Source: three-view drawing plus pictorial views. Frame: mm from the lowest corner of the part. A direction names the side the tool comes from. Coordinates: 2 decimals unless noted, no trailing zeros. Answer as a JSON object with one key per item and string values. Group by question number.
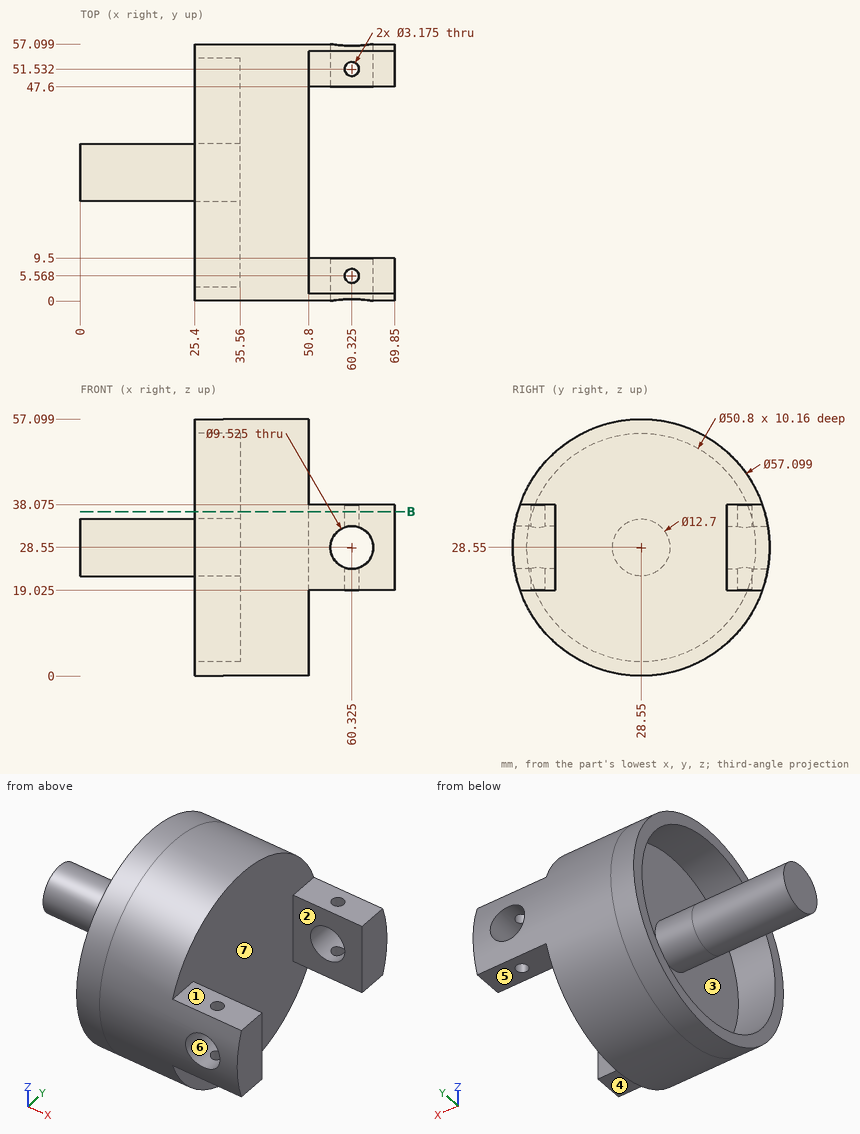
Q1. Draft query along X for the marked faces 5, 6 and 7. Return one class per face: released by +X, released by -X, zero draft, split by the parting line, or undercut.
Q2. Pin query (flat end, axial travel): pin 1 Ø8 at (y, z) = (39.5, 40.5) entering from +X; pin 2 Ø2.5 at (x, y) = (59, 4.5) entering from +Z (1 decimal); pin 3 Ø4 at (x, y) = (62, 51.5) entering from -Z (1 decimal); pin 4 Ø2.5 at (x, y) = (60.32, 51.53) entering from -Z. Return the tip coordinate at first contact, or that it passes through.
Q3. Section B-B, the plane z = 36.5. State how many separate pieces and enclosed holes the cut face has, and give its area (3 significant figures).
Q4. Line query: line 1 (X direction, y = 4, z = 41); line 2 (X direction, y = 16, z = 45); line 3 (Z direction, x = 54.5, y = 48.5) (1 decimal). Output: solid intervals per line, ascending. Write a range as from..to.
Q5. Access query for the marked faces 1, 2, 3 and 4. Directions: +Z, -Z, +X, -X, +Y, -Y. A direction counts if a zero-diameter tool reaches every point of the face in a straight line with its end or side. Return the directions, or none.
Filled in:
{
 "1": {"face 5": "zero draft", "face 6": "undercut", "face 7": "released by +X"},
 "2": {"pin 1": "x = 50.8", "pin 2": "z = 38.1", "pin 3": "z = 19", "pin 4": "through"},
 "3": {"separate pieces": "1", "enclosed holes": "2", "area": "1,210 mm^2"},
 "4": {"line 1": "25.4..50.8", "line 2": "35.56..50.8", "line 3": "19..38.1"},
 "5": {"face 1": "+Z, +X, +Y, -Y", "face 2": "+Z, -Z, +X", "face 3": "-X", "face 4": "-Z, +X, +Y, -Y"}
}
